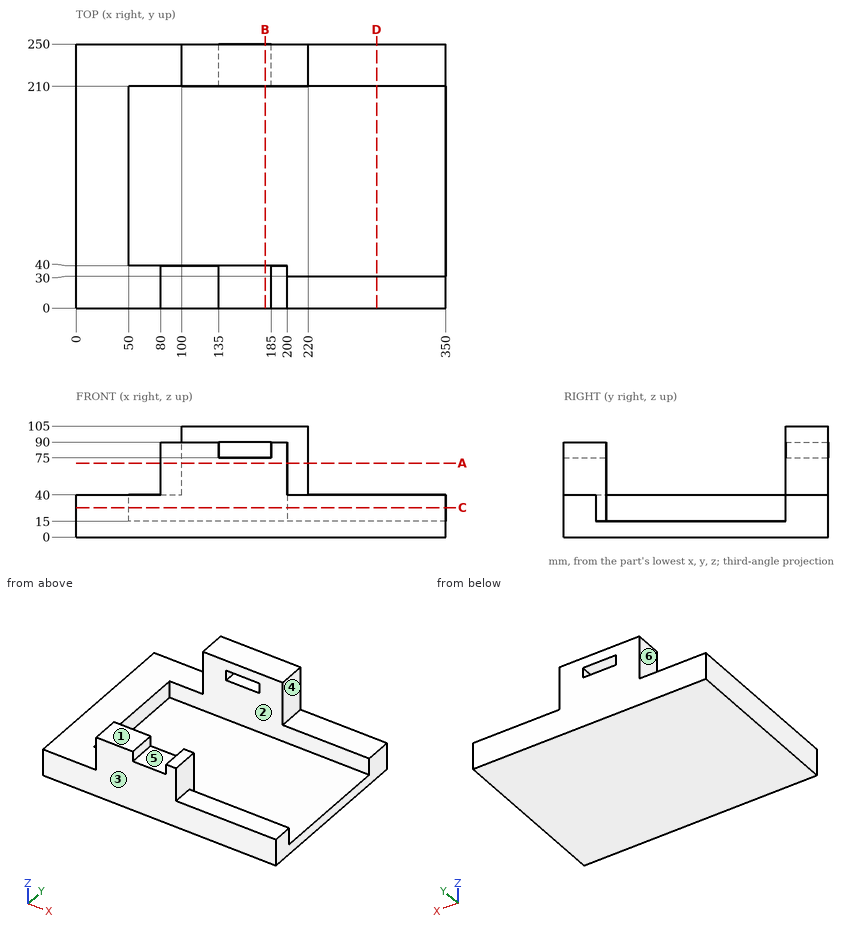
The figure shows three views and two pictorial views of one solid part (mm, origin at its lowest corner). Answer the questions. A direction names the side the tool comes from. Coordinates: 2 decimals unless noted, no trailing zeros. Loops run counter-clockwise (first coordinate to the right, second up) from the corner with the lowest first, then second, coordinate; pieces in that order, holes last. Notation, with made-up numbers: (68, -12.75) -> (116, -12.75) arc R10 ccw to (116, -3.75) -> close; hole circle Ø2 at (30, 42.25). An arc over 180 degrees is marked (long way). Write item = value, one per line. Start each with the question number.
1) Straight lines are drawn through the part: line 1 (Y direction, x = 160.5, z = 24); line 2 (Z direction, x = 28, y = 161.5); line 3 (Z direction, x = 221, y = 74). For each, find the intervals that lie inside material, in ascending order. Write a range as from..to.
2) Given pin 1 Ø12 at (x, y) = (276.5, 220.5) entering from +Z; pin 2 Ø12 at (x, y) = (193.5, 28.5) entering from +Z; pin 3 Ø12 at (y, z) = (17, 83.5) entering from -X, each flat-ended and moving along its own axis, determine where each tip first touches the part or whether it passes through.
3) A cutting plane is placed at A-A (z = 70). Give the vertices of the cut face in (x, y), then the cut area to 3 significant figures.
4) The mould has two halves that part along Y. Classify the marked faces 1, 2 and 3: released by +Y, released by -Y, zero draft, split by the parting line, or undercut.
5) A cutting plane is placed at C-C (z = 28). Give the vertices of the cut face in (x, y), then the cut area to 3 significant figures.
6) A cutting plane is placed at B-B (x = 179). Give the vertices of the cut face in (y, z), then the cut area to 3 significant figures.
7) A cutting plane is placed at D-D (x = 284.5). Give the vertices of the cut face in (y, z), then the cut area to 3 significant figures.
8) A tool of negligible diameter and unlimited length cuts with its end or side. For the marked faces 4, 5 and 6, from which of +Z, -Z, +X, -X, +Y, -Y can it reach the whole face along a straight path? Write none if from no direction.
Responses:
q1.line_1 = 0..40, 210..250
q1.line_2 = 0..40
q1.line_3 = 0..15
q2.pin_1 = 40
q2.pin_2 = 90
q2.pin_3 = 80
q3.outline = (80, 0) -> (200, 0) -> (200, 40) -> (80, 40) -> close; (100, 210) -> (220, 210) -> (220, 250) -> (100, 250) -> close
q3.area = 9,600 mm²
q4.face_1 = zero draft
q4.face_2 = undercut
q4.face_3 = released by -Y
q5.outline = (0, 0) -> (350, 0) -> (350, 30) -> (200, 30) -> (200, 40) -> (50, 40) -> (50, 210) -> (350, 210) -> (350, 250) -> (0, 250) -> close
q5.area = 35,000 mm²
q6.outline = (0, 0) -> (250, 0) -> (250, 75) -> (210, 75) -> (210, 15) -> (40, 15) -> (40, 75) -> (0, 75) -> close; (210, 90) -> (250, 90) -> (250, 105) -> (210, 105) -> close
q6.area = 9,150 mm²
q7.outline = (0, 0) -> (250, 0) -> (250, 40) -> (210, 40) -> (210, 15) -> (30, 15) -> (30, 40) -> (0, 40) -> close
q7.area = 5,500 mm²
q8.face_4 = +Z, +X, +Y, -Y
q8.face_5 = +Z, +Y, -Y
q8.face_6 = +Z, -X, +Y
